The model under review builds one solid part; all positions refer to its coordinate system, in mm. A direction names the side the tool comes from. Coordinates: 2 decimals unless noted, no trailing zeros. Loops run counter-clockwise (first coordinate to the right, second up) from the corner with the lowest first, then second, coordinate; pieces in that order, holes last. Notation, with made-up numbers: M 57.25,-36.5 L 86.25,-36.5 A23 cw 86.25,-10.5 Z; hole C 14,39.25 d1. An arc over 180 degrees is marked long. One line per item, written item: value.
```python
from build123d import *

# Parameters (mm, degrees)
BOSS_EXTRUDE1_DEPTH = 26
SKETCH2_R           = 1.5
SKETCH2_R_2         = 4
CUT_EXTRUDE1_DEPTH  = 26
FILLET1_R           = 4
SKETCH3_R           = 5
SKETCH3_R_2         = 1.5
CUT_EXTRUDE2_DEPTH  = 26


with BuildPart() as part:
    # Sketch1 → Boss-Extrude1 (new body)
    with BuildSketch(Plane.XY):
        Polygon((0, 0), (33, 0), (33, -34), (36, -34), (36, 3), (0, 3), align=None)
    extrude(amount=BOSS_EXTRUDE1_DEPTH)

    # Sketch2 → Cut-Extrude1 (cut)
    with BuildSketch(Plane(origin=(36, 0, 0), x_dir=(0, 0, -1), z_dir=(1, 0, 0))):
        with BuildLine():
            ThreePointArc((-13, -34), (-22.192388155, -30.192388155), (-26, -21))
            Line((-26, -21), (-26, -34))
            Line((-26, -34), (-13, -34))
        make_face()
        with BuildLine():
            ThreePointArc((0, -21), (-3.807611845, -30.192388155), (-13, -34))
            Line((-13, -34), (0, -34))
            Line((0, -34), (0, -21))
        make_face()
        with Locations((-4.5, -21)):
            Circle(SKETCH2_R)
        with Locations((-13, -21)):
            Circle(SKETCH2_R_2)
        with Locations((-21.5, -21)):
            Circle(SKETCH2_R)
    extrude(amount=-CUT_EXTRUDE1_DEPTH, mode=Mode.SUBTRACT)

    # Fillet1
    fillet1_edges = [part.edges().sort_by_distance(p)[0] for p in [
        (36, 3, 13),
        (33, 0, 13),
    ]]
    fillet(fillet1_edges, radius=FILLET1_R)

    # Sketch3 → Cut-Extrude2 (cut)
    with BuildSketch(Plane(origin=(0, 3, 0), x_dir=(1, 0, 0), z_dir=(0, 1, 0))):
        with Locations((15, -13)):
            Circle(SKETCH3_R)
        with Locations((23, -21)):
            Circle(SKETCH3_R_2)
        with Locations((23, -5)):
            Circle(SKETCH3_R_2)
        with Locations((7, -5)):
            Circle(SKETCH3_R_2)
        with Locations((7, -21)):
            Circle(SKETCH3_R_2)
    extrude(amount=-CUT_EXTRUDE2_DEPTH, mode=Mode.SUBTRACT)


solid = part.part
```
(1) Add section A-A on y = -24. State the section outline as (x, z) points, then the cut area to 3 significant figures.
Checks:
outline: M 33,0.35 L 36,0.35 L 36,10.35 L 33,10.35 Z; M 33,15.65 L 36,15.65 L 36,25.65 L 33,25.65 Z
area: 60.0 mm^2
(2) To check wall thickness, follow L1, parallel to X at y = 1.15, z = 21; L2, parallel to Z at x = 15, y = 1; L3, parallel to X at y = 1, z = 6.25. State the ranges of each line that lie inside material, in increasing order. Write a range as [from, to].
Checks:
L1: [0, 5.5], [8.5, 21.5], [24.5, 35.37]
L2: [0, 8], [18, 26]
L3: [0, 6.17], [7.83, 22.17], [23.83, 35.46]
(3) Add section D-D on x = 12.5. State the section outline as (y, z) points, then the cut area to 3 significant figures.
Checks:
outline: M 0,0 L 3,0 L 3,8.67 L 0,8.67 Z; M 0,17.33 L 3,17.33 L 3,26 L 0,26 Z
area: 52.0 mm^2
(4) Tool access review of faces 4 (the face through (33, -15, 13)), 5 (the face through (34.797, 1.859, 13.182)): name each direction out of +Z, -Z, +X, -X, +Y, -Y from which nothing blocks a thin tool from reaching the whole face with its end or side.
Checks:
face 4: +Z, -Z, -X, -Y
face 5: +Z, -Z, +X, +Y
(5) Insertion check: pin 1 Ø2.5 at (x, z) = (23, 21) entering from +Y; pin 2 Ø5 at (x, z) = (7, 21) entering from -Y; pin 3 Ø12 at (x, z) = (25, 6.5) entering from -Y. Each pin has a flat end and moves straight along its axis. Give the tip position at first contact, or say it passes through.
Checks:
pin 1: through
pin 2: y = 0
pin 3: y = -0.54
(6) Add section B-B on x = 23. State the section outline as (y, z) points, then the cut area to 3 significant figures.
Checks:
outline: M 0,0 L 3,0 L 3,3.5 L 0,3.5 Z; M 0,6.5 L 3,6.5 L 3,19.5 L 0,19.5 Z; M 0,22.5 L 3,22.5 L 3,26 L 0,26 Z
area: 60.0 mm^2
(7) Add section C-C on z = 4.5. State the section outline as (x, y) points, then the cut area to 3 significant figures.
Checks:
outline: M 0,0 L 5.59,0 L 5.59,3 L 0,3 Z; M 8.41,0 L 21.59,0 L 21.59,3 L 8.41,3 Z; M 24.41,0 L 29,0 A4 cw 33,-4 L 33,-19.5 L 36,-19.5 L 36,-1 A4 ccw 32,3 L 24.41,3 Z; M 33,-30.84 L 36,-30.84 L 36,-22.5 L 33,-22.5 Z
area: 175 mm^2
(8) Draft analysis for pull direction Z (two halves, no side actions). For faces 1 (the face through (14, 0, 7)), 2 (the face through (5.5, 1.52, 4.93)), 3 (the face through (25, 1, 26)), state which applies: pulls with the +Z half, pulls with the -Z half, needs draft (parallel to the pull), parting line crosses it, or undercut.
Checks:
face 1: needs draft
face 2: undercut
face 3: pulls with the +Z half
